from build123d import *

# Parameters (mm, degrees)
EXTRUDE1_DEPTH     = 3.25
SKETCH2_W          = 1.75
SKETCH2_H          = 1.75
SKETCH2_H_2        = 1.6
SKETCH2_H_3        = 0.6
CUT_EXTRUDE1_DEPTH = 2.65
CUT_EXTRUDE3_DEPTH = 1.75
CUT_EXTRUDE4_DEPTH = 1.75


with BuildPart() as part:
    # Sketch1 → Extrude1 (new body, symmetric)
    with BuildSketch(Plane.XY):
        with BuildLine():
            Line((-1.640721741, 0.89), (1.640721741, 0.89))
            Line((1.640721741, 0.89), (1.75, 0))
            Line((1.75, 0), (1.977970995, 0))
            ThreePointArc((1.977970995, 0), (2.180892756, -0.043028711), (2.34888867, -0.164708965))
            Line((2.34888867, -0.164708965), (2.586570168, -0.427645517))
            ThreePointArc((2.586570168, -0.427645517), (2.670568125, -0.488485644), (2.772029005, -0.51))
            Line((2.772029005, -0.51), (3.5, -0.51))
            Line((3.5, -0.51), (3.5, -0.76))
            Line((3.5, -0.76), (2.772029005, -0.76))
            ThreePointArc((2.772029005, -0.76), (2.569107244, -0.716971289), (2.40111133, -0.595291035))
            Line((2.40111133, -0.595291035), (2.163429832, -0.332354483))
            ThreePointArc((2.163429832, -0.332354483), (2.079431875, -0.271514356), (1.977970995, -0.25))
            Line((1.977970995, -0.25), (1.75, -0.25))
            Line((1.75, -0.25), (1.693519102, -0.71))
            Line((1.693519102, -0.71), (-1.693519102, -0.71))
            Line((-1.693519102, -0.71), (-1.75, -0.25))
            Line((-1.75, -0.25), (-1.977970995, -0.25))
            ThreePointArc((-1.977970995, -0.25), (-2.079431875, -0.271514356), (-2.163429832, -0.332354483))
            Line((-2.163429832, -0.332354483), (-2.40111133, -0.595291035))
            ThreePointArc((-2.40111133, -0.595291035), (-2.569107244, -0.716971289), (-2.772029005, -0.76))
            Line((-2.772029005, -0.76), (-3.5, -0.76))
            Line((-3.5, -0.76), (-3.5, -0.51))
            Line((-3.5, -0.51), (-2.772029005, -0.51))
            ThreePointArc((-2.772029005, -0.51), (-2.670568125, -0.488485644), (-2.586570168, -0.427645517))
            Line((-2.586570168, -0.427645517), (-2.34888867, -0.164708965))
            ThreePointArc((-2.34888867, -0.164708965), (-2.180892756, -0.043028711), (-1.977970995, 0))
            Line((-1.977970995, 0), (-1.75, 0))
            Line((-1.75, 0), (-1.640721741, 0.89))
        make_face()
    extrude(amount=EXTRUDE1_DEPTH, both=True)

    # Sketch2 → Cut-Extrude1 (cut, through all)
    with BuildSketch(Plane(origin=(0, 0.89, 0), x_dir=(1, 0, 0), z_dir=(0, 1, 0))):
        with Locations((-2.625, 2.375)):
            Rectangle(SKETCH2_W, SKETCH2_H)
        with Locations((-2.625, -2.375)):
            Rectangle(SKETCH2_W, SKETCH2_H)
        with Locations((2.625, 1.15)):
            Rectangle(SKETCH2_W, SKETCH2_H_2)
        with Locations((2.625, -1.15)):
            Rectangle(SKETCH2_W, SKETCH2_H_2)
        with Locations((2.625, 2.95)):
            Rectangle(SKETCH2_W, SKETCH2_H_3)
        with Locations((2.625, -2.95)):
            Rectangle(SKETCH2_W, SKETCH2_H_3)
    extrude(amount=-CUT_EXTRUDE1_DEPTH, mode=Mode.SUBTRACT)

    # Sketch3 → Cut-Extrude3 (cut, symmetric)
    with BuildSketch(Plane(origin=(0, 0, 0), x_dir=(0, 0, -1), z_dir=(1, 0, 0))):
        Polygon((3.140721741, 0.89), (3.25, 0), (3.25, 0.89), align=None)
        Polygon((-3.25, 0), (-3.25, 0.89), (-3.140721741, 0.89), align=None)
    extrude(amount=CUT_EXTRUDE3_DEPTH, both=True, mode=Mode.SUBTRACT)

    # Sketch4 → Cut-Extrude4 (cut, symmetric)
    with BuildSketch(Plane(origin=(0, 0, 0), x_dir=(0, 0, -1), z_dir=(1, 0, 0))):
        Polygon((3.162822962, -0.71), (3.25, -0.71), (3.25, 0), align=None)
        Polygon((-3.25, 0), (-3.162822962, -0.71), (-3.25, -0.71), align=None)
    extrude(amount=CUT_EXTRUDE4_DEPTH, both=True, mode=Mode.SUBTRACT)


solid = part.part
Could you check a few things on this model? Use its own coordinates, in mm. A direction names the side the tool comes from. Give positions to 0.01 mm unless a question says otherwise; leave off trailing zeros. Order: outer loops, then holes, each group sorted by start corner. A loop starts at its lowest first (then second) coordinate and runs counter-clockwise, first axis right, second up.
1. Suppose I cut it at D-D (z = -0.25). List the corners of the cut face in (x, y) for me.
2. Will these pins go through, and if not, where does the flat tip stop? P1, Ø3, axis at x = 1, z = 2.5, coming from the -Y side; P2, Ø0.8, axis at x = 2.5, y = 0, coming from the -Z side.
3. For faces 1 (the flat face through (0, -0.71, 0)), 2 (the flat face through (0, 0.89, 0)), which set-ups out of +Z, -Z, +X, -X, +Y, -Y let a thin tool reach every point of the face, with its end or its side?
4. Suppose I cut it at A-A (z = 2.25). List the corners of the cut face in (x, y) for me, plus the area to 3 significant figures.
5. Suppose I cut it at C-C (y = 0.1). List the corners of the cut face in (x, z) for me.
6. I need wall thicknesses on L1, parallel to Y at x = 1.25, z = -2.5; L2, parallel to Y at x = -2, z = 0.5; L3, parallel to X at y = 0.45, z = 2.25. Which ranges of each line are inside material? Lowest first, please.
7. Suppose I cut it at B-B (x = -1.25). List the corners of the cut face in (y, z) for me, plus the area to 3 significant figures.
Solved:
1. outline: (-3.5, -0.76) - (-2.77, -0.76) arc R0.5 ccw to (-2.4, -0.6) - (-2.16, -0.33) arc R0.25 cw to (-1.98, -0.25) - (-1.75, -0.25) - (-1.69, -0.71) - (1.69, -0.71) - (1.75, -0.25) - (1.98, -0.25) arc R0.25 cw to (2.16, -0.33) - (2.4, -0.6) arc R0.5 ccw to (2.77, -0.76) - (3.5, -0.76) - (3.5, -0.51) - (2.77, -0.51) arc R0.25 cw to (2.59, -0.43) - (2.35, -0.16) arc R0.5 ccw to (1.98, 0) - (1.75, 0) - (1.64, 0.89) - (-1.64, 0.89) - (-1.75, 0) - (-1.98, 0) arc R0.5 ccw to (-2.35, -0.16) - (-2.59, -0.43) arc R0.25 cw to (-2.77, -0.51) - (-3.5, -0.51) - close
2. P1: stops at y = -0.71
2. P2: stops at z = -2.65
3. face 1: +Z, -Z, -Y
3. face 2: +Z, -Z, +X, -X, +Y
4. outline: (-1.75, -0.25) - (-1.69, -0.71) - (1.69, -0.71) - (1.75, -0.25) - (1.98, -0.25) arc R0.25 cw to (2.16, -0.33) - (2.4, -0.6) arc R0.5 ccw to (2.77, -0.76) - (3.5, -0.76) - (3.5, -0.51) - (2.77, -0.51) arc R0.25 cw to (2.59, -0.43) - (2.35, -0.16) arc R0.5 ccw to (1.98, 0) - (1.75, 0) - (1.64, 0.89) - (-1.64, 0.89) - (-1.75, 0) - close
4. area: 5.96 mm2
5. outline: (-1.74, -3.24) - (1.74, -3.24) - (1.74, 3.24) - (-1.74, 3.24) - close
6. L1: y = -0.71 to 0.89
6. L2: y = -0.25 to 0
6. L3: x = -1.69 to 1.69
7. outline: (-0.71, -3.16) - (0, -3.25) - (0.89, -3.14) - (0.89, 3.14) - (0, 3.25) - (-0.71, 3.16) - close
7. area: 10.2 mm2
